Design review of the part built by this model. Coordinates are the model's own, in mm. A direction names the side the tool comes from. Give positions to 0.01 mm unless a question says otherwise; leave off trailing zeros. Write each loop counter-clockwise with the first axis right and the second up, starting at its lowest first coordinate (ties: lowest second). Pieces come first, ordered by that corner, then holes. Notation, with made-up numbers: M 74.25,3.5 L 127.25,3.5 A17 ccw 127.25,31.5 Z; hole C 41.25,69 d2. An arc over 180 degrees is marked long. Use one line per item in the form item = value. Start each with the question number.
from build123d import *

# Parameters (mm, degrees)
BODY_EXTRUDE_DEPTH              = 12
M4X0_7_TAPPED_HOLE6_D           = 3.3
M4X0_7_TAPPED_HOLE6_CSINK_D     = 4.05
M4X0_7_TAPPED_HOLE6_CSINK_ANGLE = 90
CUT_EXTRUDE1_DEPTH              = 32.10064308
CHAMFER1_SIZE                   = 1


with BuildPart() as part:
    # Sketch1 → Body Extrude (new body)
    with BuildSketch(Plane.XY):
        Polygon((-26.5, 0), (26.5, 0), (26.5, 5), (4.5, 5), (4.5, 11), (-4.5, 11), (-4.5, 5), (-26.5, 5), align=None)
    extrude(amount=-BODY_EXTRUDE_DEPTH)

    # M4x0.7 Tapped Hole6 (through all)
    with Locations(Plane.XZ):
        with Locations((-22.5, -6), (22.5, -6)):
            CounterSinkHole(M4X0_7_TAPPED_HOLE6_D / 2, M4X0_7_TAPPED_HOLE6_CSINK_D / 2, counter_sink_angle=M4X0_7_TAPPED_HOLE6_CSINK_ANGLE)

    # Sketch2 → Cut-Extrude1 (cut, through all)
    with BuildSketch(Plane(origin=(0, 0, 0), x_dir=(1, 0, 0), z_dir=(0, 1, 0))):
        with BuildLine():
            Line((-1.581929202, 4), (1.581929202, 4))
            ThreePointArc((1.581929202, 4), (0, 8.55), (-1.581929202, 4))
        make_face()
    extrude(amount=CUT_EXTRUDE1_DEPTH, mode=Mode.SUBTRACT)

    # Chamfer1
    chamfer1_edges = [part.edges().sort_by_distance(p)[0] for p in [
        (26.5, 2.5, 0),
        (-26.5, 2.5, 0),
        (26.5, 2.5, -12),
        (-26.5, 2.5, -12),
    ]]
    chamfer(chamfer1_edges, length=CHAMFER1_SIZE)


solid = part.part
1. Draft analysis for pull direction Z (two halves, no side actions). For faces 6 (the flat face through (-26, 2.5, -0.5)), 7 (the cylindrical face through (24.15, 2.72, -5.93)), 8 (the flat face through (-26.5, 3, -6)), state which applies: pulls with the +Z half, pulls with the -Z half, needs draft (parallel to the pull), parting line crosses it, or undercut.
2. Clearance check with flat-ended pins moving along their axes: pin 1 Ø6.5 at (y, z) = (9, -4) entering from +X; pin 2 Ø5 at (x, z) = (19.5, -3.5) entering from +Y; pin 3 Ø5 at (y, z) = (8.5, -7.5) entering from -X. State where each tip first meets the part, or that it passes through.
3. We need section A-A (z = -6). State the section outline as (x, y) points (3 decimals).
4. For faces 1 (the flat face through (0, 5, -4)), 2 (the flat face through (-4.5, 8, -6)), 3 (the flat face through (0, 3, 0)), 4 (the flat face through (4.5, 8, -6)), 5 (the flat face through (0, 11, -3)), list the 3-axis set-ups (+Z, -Z, +X, -X, +Y, -Y) from which the entire face can be reached by the end or side of a thin tool; tool diameter is ignored.
5. We need section D-D (y = 1.75). State the section outline as (x, z) points.
6. We need section B-B (x = 22.5). State the section outline as (y, z) points (3 decimals).
7. To check wall thickness, follow L1, parallel to X at y = 4, z = -6; L2, parallel to Z at x = 22.5, y = 3; L3, parallel to Z at x = 0, y = 4.5. State the ranges of each line that lie inside material, in increasing order.
8. We need section C-C (y = 6.5). State the section outline as (x, z) points.
Answer block:
q1.face_6 = pulls with the +Z half
q1.face_7 = undercut
q1.face_8 = needs draft
q2.pin_1 = 4.5
q2.pin_2 = 5
q2.pin_3 = -4.5
q3.outline = M -26.5,0 L -24.525,0 L -24.15,0.375 L -24.15,5 L -26.5,5 Z; M -20.85,0.375 L -20.475,0 L -2.55,0 L -2.55,11 L -4.5,11 L -4.5,5 L -20.85,5 Z; M 2.55,0 L 20.475,0 L 20.85,0.375 L 20.85,5 L 4.5,5 L 4.5,11 L 2.55,11 Z; M 24.15,0.375 L 24.525,0 L 26.5,0 L 26.5,5 L 24.15,5 Z
q4.face_1 = +Y, -Y
q4.face_2 = +Z, -Z, -X, +Y
q4.face_3 = +Z, +X, -X, +Y, -Y
q4.face_4 = +Z, -Z, +X, +Y
q4.face_5 = +Z, -Z, +X, -X, +Y
q5.outline = M -26.5,-11 L -25.5,-12 L 25.5,-12 L 26.5,-11 L 26.5,-1 L 25.5,0 L -25.5,0 L -26.5,-1 Z; hole C -22.5,-6 d3.3; hole M -1.58,-4 A2.55 ccw long 1.58,-4 Z; hole C 22.5,-6 d3.3
q6.outline = M 0,-12 L 5,-12 L 5,-7.65 L 0.375,-7.65 L 0,-8.025 Z; M 0,-3.975 L 0.375,-4.35 L 5,-4.35 L 5,0 L 0,0 Z
q7.L1 = -26.5 to -24.15, -20.85 to -2.55, 2.55 to 20.85, 24.15 to 26.5
q7.L2 = -12 to -7.65, -4.35 to 0
q7.L3 = -12 to -8.55, -4 to 0
q8.outline = M -4.5,-12 L 4.5,-12 L 4.5,0 L -4.5,0 Z; hole M -1.58,-4 A2.55 ccw long 1.58,-4 Z
